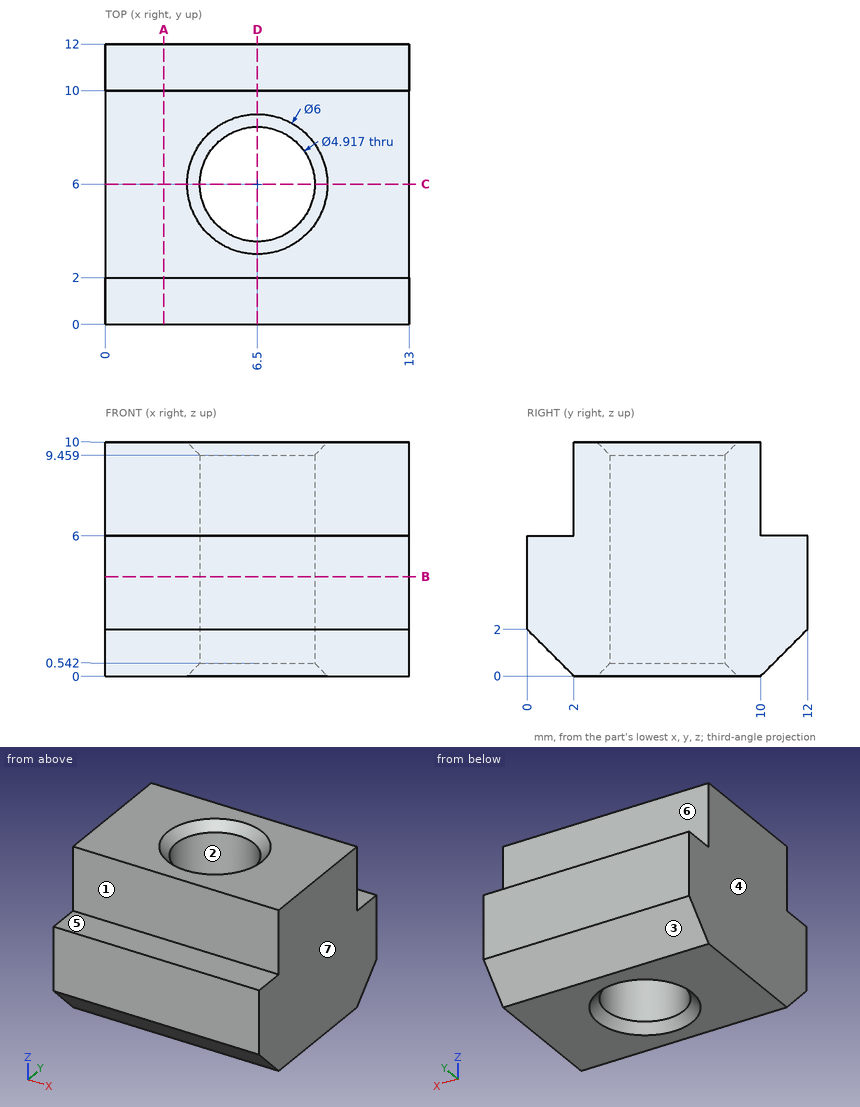
Study the drawing (mm; zero at the part's minimum x, y, z) and answer. A direction names the side the tool comes from. Coordinates: 2 decimals unless noted, no trailing zeros. Write each loop counter-clockwise with the first axis right and the second up, starting at its lowest first coordinate (ties: lowest second). Pieces come first, ordered by that corner, then holes. Notation, with made-up numbers: (48.5, -33.5) - (66.5, -33.5) arc R13 cw to (66.5, -16.5) - close; hole circle Ø2 at (-20.75, 12). An arc over 180 degrees is marked (long way). Answer as a JSON object with one key per item and string values. Group by question number.
1. A cutting plane is placed at D-D (x = 6.5). Determine the outline of the cut face in (y, z).
2. Each of these flat-tipped pins is pushed along its axis until it touches: P1, Ø1, axis at x = 8.5, y = 11, coming from the +Z side; P2, Ø3, axis at x = 9.5, z = 8, coming from the -Y side. Where does it stop, or does it pass through?
3. A cutting plane is placed at B-B (z = 4.25). Determine the outline of the cut face in (x, y).
4. Consider L1, parallel to Y at x = 6.5, z = 7; L2, parallel to X at y = 6, z = 4; L3, parallel to Y at x = 11, z = 8. Determine where each line is inside the solid, lowest interval first. Write a range as [from, to].
5. A cutting plane is placed at A-A (x = 2.5). Determine the outline of the cut face in (y, z).
6. A cutting plane is placed at C-C (y = 6). Determine the outline of the cut face in (x, z).
7. Which of the six approach directions +Z, -Z, +X, -X, +Y, -Y give full straight-line access (tool end or side, diameter ignored) to the marked faces 5, 6 and 7?
8. The mould has two halves that part along Y. Classify the marked faces 1, 2, 3 and 4: +Y half, -Y half, draft (parallel to the pull), parting line (faces both ways), or undercut.
Worked out:
{
 "1": {"outline": "(0, 2) - (2, 0) - (3, 0) - (3.54, 0.54) - (3.54, 9.46) - (3, 10) - (2, 10) - (2, 6) - (0, 6) - close; (8.46, 0.54) - (9, 0) - (10, 0) - (12, 2) - (12, 6) - (10, 6) - (10, 10) - (9, 10) - (8.46, 9.46) - close"},
 "2": {"P1": "stops at z = 6", "P2": "stops at y = 2"},
 "3": {"outline": "(0, 0) - (13, 0) - (13, 12) - (0, 12) - close; hole circle Ø4.92 at (6.5, 6)"},
 "4": {"L1": "y = [2, 3.54], [8.46, 10]", "L2": "x = [0, 4.04], [8.96, 13]", "L3": "y = [2, 10]"},
 "5": {"outline": "(0, 2) - (2, 0) - (10, 0) - (12, 2) - (12, 6) - (10, 6) - (10, 10) - (2, 10) - (2, 6) - (0, 6) - close"},
 "6": {"outline": "(0, 0) - (3.5, 0) - (4.04, 0.54) - (4.04, 9.46) - (3.5, 10) - (0, 10) - close; (8.96, 0.54) - (9.5, 0) - (13, 0) - (13, 10) - (9.5, 10) - (8.96, 9.46) - close"},
 "7": {"face 5": "+Z, +X, -X, -Y", "face 6": "+Z, +X, -X, +Y", "face 7": "+Z, -Z, +X, +Y, -Y"},
 "8": {"face 1": "-Y half", "face 2": "undercut", "face 3": "+Y half", "face 4": "draft"}
}
